Could you check a few things on this model? Use its own coordinates, in mm. A direction names the side the tool comes from. Coordinates: 2 decimals unless noted, no trailing zeros.
```python
from build123d import *

# Parameters (mm, degrees)
BOX001_W        = 38.73
BOX001_H        = 53.34
BOX001_DEPTH    = 50.8
SKETCH_W        = 139.7
SKETCH_H        = 127
SKETCH_W_2      = 130.175
SKETCH_H_2      = 115.8875
PAD_DEPTH       = 31.75
SKETCH001_W     = 139.7
SKETCH001_H     = 127
SKETCH001_R     = 1.651
PAD001_DEPTH    = 4.7625
SKETCH002_R     = 5.08
SKETCH002_R_2   = 2.286
PAD002_DEPTH    = 31.75
SKETCH003_W     = 25.4
SKETCH003_H     = 40
PAD003_DEPTH    = 24.5
POCKET_DEPTH    = 139.701
SKETCH007_R     = 4.445
SKETCH007_R_2   = 1.45
PAD006_DEPTH    = 6.35
SKETCH014_R     = 1.905
POCKET004_DEPTH = 6.351
SKETCH015_W     = 133.35
SKETCH015_H     = 120.65
POCKET005_DEPTH = 6.35
SKETCH016_R     = 1.651
PAD010_DEPTH    = 3.175
SKETCH060_W     = 10.16
SKETCH060_H     = 9.525
SKETCH060_W_2   = 7.62
SKETCH060_H_2   = 1.143
PAD028_DEPTH    = 9.525
SKETCH061_R     = 1.6
POCKET028_DEPTH = 11.43
SKETCH071_W     = 4.522567
SKETCH071_H     = 19.0781560115
PAD033_DEPTH    = 28.575
SKETCH072_R     = 1.778
POCKET034_DEPTH = 76.2
SKETCH074_W     = 4.299609
SKETCH074_H     = 32.990636
SKETCH074_W_2   = 34.861665
SKETCH074_H_2   = 4.058911
PAD034_DEPTH    = 28.575
SKETCH089_W     = 5.08
SKETCH089_H     = 47.5033603219
SKETCH089_R     = 1.45
PAD041_DEPTH    = 19.05


with BuildPart() as front_removal:
    # Box001 → Box001 (new body)
    with BuildSketch(Plane(origin=(-14.6558, 22.7838, 0), x_dir=(1, 0, 0), z_dir=(0, 0, 1))):
        with Locations((19.365, 26.67)):
            Rectangle(BOX001_W, BOX001_H)
    extrude(amount=BOX001_DEPTH)


with BuildPart() as main_body:
    # Sketch → Pad (new body)
    with BuildSketch(Plane.XY):
        Rectangle(SKETCH_W, SKETCH_H)
        with Locations((0, -0.79375)):
            Rectangle(SKETCH_W_2, SKETCH_H_2, mode=Mode.SUBTRACT)
    extrude(amount=PAD_DEPTH)

    # Sketch001 (on Face9 of Pad) → Pad001 (join)
    with BuildSketch(Plane(origin=(0, 0, 0), x_dir=(1, 0, 0), z_dir=(0, 0, -1))):
        Rectangle(SKETCH001_W, SKETCH001_H)
        with Locations((-27.286566, 13.226975)):
            Circle(SKETCH001_R, mode=Mode.SUBTRACT)
        with Locations((-27.286566, -2.648025)):
            Circle(SKETCH001_R, mode=Mode.SUBTRACT)
        with Locations((-9.8298, -32.495678)):
            Circle(SKETCH001_R, mode=Mode.SUBTRACT)
        with Locations((19.2024, -32.495678)):
            Circle(SKETCH001_R, mode=Mode.SUBTRACT)
        with Locations((19.2024, -56.625678)):
            Circle(SKETCH001_R, mode=Mode.SUBTRACT)
        with Locations((-9.8298, -56.625678)):
            Circle(SKETCH001_R, mode=Mode.SUBTRACT)
    extrude(amount=PAD001_DEPTH)

    # Sketch002 (on Face21 of Pad001) → Pad002 (join)
    with BuildSketch(Plane.XY):
        with Locations((-62.70625, 55.5625)):
            Circle(SKETCH002_R)
        with Locations((-62.70625, 55.5625)):
            Circle(SKETCH002_R_2, mode=Mode.SUBTRACT)
        with Locations((0, 55.5625)):
            Circle(SKETCH002_R)
        with Locations((0, 55.5625)):
            Circle(SKETCH002_R_2, mode=Mode.SUBTRACT)
        with Locations((62.70625, 55.5625)):
            Circle(SKETCH002_R)
        with Locations((62.70625, 55.5625)):
            Circle(SKETCH002_R_2, mode=Mode.SUBTRACT)
        with Locations((62.70625, 0)):
            Circle(SKETCH002_R)
        with Locations((62.70625, 0)):
            Circle(SKETCH002_R_2, mode=Mode.SUBTRACT)
        with Locations((62.70625, -55.5625)):
            Circle(SKETCH002_R)
        with Locations((62.70625, -55.5625)):
            Circle(SKETCH002_R_2, mode=Mode.SUBTRACT)
        with Locations((0, -55.5625)):
            Circle(SKETCH002_R)
        with Locations((0, -55.5625)):
            Circle(SKETCH002_R_2, mode=Mode.SUBTRACT)
        with Locations((-62.70625, -55.5625)):
            Circle(SKETCH002_R)
        with Locations((-62.70625, -55.5625)):
            Circle(SKETCH002_R_2, mode=Mode.SUBTRACT)
        with Locations((-62.70625, 0)):
            Circle(SKETCH002_R)
        with Locations((-62.70625, 0)):
            Circle(SKETCH002_R_2, mode=Mode.SUBTRACT)
    extrude(amount=PAD002_DEPTH)

    # Sketch003 (on Face33 of Pad002) → Pad003 (join)
    with BuildSketch(Plane.XY):
        with Locations((-57.15, -33.97)):
            Rectangle(SKETCH003_W, SKETCH003_H)
        with Locations((57.15, -33.97)):
            Rectangle(SKETCH003_W, SKETCH003_H)
    extrude(amount=PAD003_DEPTH)

    # Sketch004 (on Face7 of Pad003) → Pocket (cut, through all)
    with BuildSketch(Plane(origin=(-69.85, 0, 0), x_dir=(0, -1, 0), z_dir=(-1, 0, 0))):
        with BuildLine():
            ThreePointArc((24.511, 20.5930335595), (34.036, 0), (43.561, 20.5930335595))
            Line((43.561, 33.2930335595), (43.561, 20.5930335595))
            Line((24.511, 33.2930335595), (43.561, 33.2930335595))
            Line((24.511, 20.5930335595), (24.511, 33.2930335595))
        make_face()
    extrude(amount=-POCKET_DEPTH, mode=Mode.SUBTRACT)

    # Sketch007 → Pad006 (join)
    with BuildSketch(Plane(origin=(-34.29, 25.4, 0), x_dir=(1, 0, 0), z_dir=(0, 0, 1))):
        with Locations((5.08, 23.11)):
            Circle(SKETCH007_R)
        with Locations((5.08, 23.11)):
            Circle(SKETCH007_R_2, mode=Mode.SUBTRACT)
        with Locations((-26.92, 23.11)):
            Circle(SKETCH007_R)
        with Locations((-26.92, 23.11)):
            Circle(SKETCH007_R_2, mode=Mode.SUBTRACT)
        with Locations((-26.92, -8.89)):
            Circle(SKETCH007_R)
        with Locations((-26.92, -8.89)):
            Circle(SKETCH007_R_2, mode=Mode.SUBTRACT)
        with Locations((5.08, -8.89)):
            Circle(SKETCH007_R)
        with Locations((5.08, -8.89)):
            Circle(SKETCH007_R_2, mode=Mode.SUBTRACT)
    extrude(amount=PAD006_DEPTH)

    # Sketch014 (on Face19 of Pad006) → Pocket004 (cut, through all)
    with BuildSketch(Plane.XZ.offset(-57.15)):
        with Locations((-47.625, 21.59)):
            Circle(SKETCH014_R)
        with Locations((-28.575, 15.24)):
            Circle(SKETCH014_R)
        with Locations((33.655, 15.24)):
            Circle(SKETCH014_R)
        with Locations((52.705, 21.59)):
            Circle(SKETCH014_R)
    extrude(amount=-POCKET004_DEPTH, mode=Mode.SUBTRACT)

    # Sketch015 → Pocket005 (cut)
    with BuildSketch(Plane.XY.offset(29.21)):
        Rectangle(SKETCH015_W, SKETCH015_H)
    extrude(amount=POCKET005_DEPTH, mode=Mode.SUBTRACT)

    # Sketch016 (on Face11 of Pocket005) → Pad010 (join)
    with BuildSketch(Plane(origin=(-69.85, 0, 0), x_dir=(0, -1, 0), z_dir=(-1, 0, 0))):
        with BuildLine():
            ThreePointArc((30.226, 12.3860423935), (34.036, 8.5760423935), (37.846, 12.3860423935))
            Line((43.561, 20.5930335595), (37.846, 12.3860423935))
            ThreePointArc((24.511, 20.5930335595), (34.036, -0.1869576065), (43.561, 20.5930335595))
            Line((24.511, 20.5930335595), (30.226, 12.3860423935))
        make_face()
        with Locations((25.536, 12.49934)):
            Circle(SKETCH016_R, mode=Mode.SUBTRACT)
        with Locations((42.536, 12.49934)):
            Circle(SKETCH016_R, mode=Mode.SUBTRACT)
    pad010 = extrude(amount=-PAD010_DEPTH)

    # Mirrored: Pad010 across YZ
    add(pad010.mirror(Plane.YZ))

    # Sketch060 (on Face81 of Pocket005) → Pad028 (join)
    with BuildSketch(Plane.XY):
        with Locations((17.78, -53.975)):
            Rectangle(SKETCH060_W, SKETCH060_H)
        with Locations((17.78, -52.2605)):
            Rectangle(SKETCH060_W_2, SKETCH060_H_2, mode=Mode.SUBTRACT)
        with Locations((17.78, -56.5785)):
            Rectangle(SKETCH060_W_2, SKETCH060_H_2, mode=Mode.SUBTRACT)
    extrude(amount=PAD028_DEPTH)

    # Sketch061 (on Face86 of Pad028) → Pocket028 (cut)
    with BuildSketch(Plane.XZ.offset(63.5)):
        with Locations((17.78, 5.08)):
            Circle(SKETCH061_R)
    extrude(amount=-POCKET028_DEPTH, mode=Mode.SUBTRACT)

    # Sketch071 (on Face21 of Pad001) → Pad033 (join)
    with BuildSketch(Plane.XY):
        with Locations((-16.9815035, 50.9765749943)):
            Rectangle(SKETCH071_W, SKETCH071_H)
        with Locations((26.3779375001, 50.9765749943)):
            Rectangle(SKETCH071_W, SKETCH071_H)
    extrude(amount=PAD033_DEPTH)

    # Sketch072 (on Face127 of Pad033) → Pocket034 (cut)
    with BuildSketch(Plane.XY.offset(31.75)):
        with Locations((50.8, 22.225)):
            Circle(SKETCH072_R)
    extrude(amount=-POCKET034_DEPTH, mode=Mode.SUBTRACT)

    # Sketch074 (on Face56 of Pocket034) → Pad034 (join)
    with BuildSketch(Plane.XY):
        with Locations((-17.2816815, 25.842361)):
            Rectangle(SKETCH074_W, SKETCH074_H)
        with Locations((2.0425745, -22.9079595)):
            Rectangle(SKETCH074_W_2, SKETCH074_H_2)
    extrude(amount=PAD034_DEPTH)

    # Sketch089 (on Face56 of Pad034) → Pad041 (join)
    with BuildSketch(Plane.XY):
        with Locations((26.6647168511, 17.7529041609)):
            Rectangle(SKETCH089_W, SKETCH089_H)
        with Locations((26.6647168511, 32.117611)):
            Circle(SKETCH089_R, mode=Mode.SUBTRACT)
        with Locations((26.6647168511, 6.717611)):
            Circle(SKETCH089_R, mode=Mode.SUBTRACT)
    extrude(amount=PAD041_DEPTH)

    # Cut001: cut front-removal
    add(front_removal.part, mode=Mode.SUBTRACT)


solid = main_body.part
```
Item 1: Thinking about a two-plate mould opening in Y: for faces 1 (the face through (-10.188, 58.237, -2.348)), 2 (the face through (-67, 33, 31.75)), which applies, +Y half, -Y half, draft (parallel to the pull), parting line (faces both ways), or undercut?
Item 2: I need wall thicknesses on line 1 (X direction, y = 31, z = 23.5); line 2 (X direction, y = 28, z = 4); line 3 (Y direction, x = -22.5, z = 5). Which ranges of each line are inside material? Lowest first, please.
Item 3: For pin 1 Ø1 at (x, z) = (-2, 8.5) entering from +Y; pin 2 Ø1.7 at (x, y) = (26.66, 6.72) entering from +Z; pin 3 Ø3.5 at (x, y) = (-62.71, 55.56) entering from +Z, each with a flat end and sliding along its axis, tell me the tip position at first contact or that it passes through.
Item 4: Which directions (+Z, -Z, +X, -X, +Y, -Y) give clear straight access to the entire face, cutting with the end or side of a thin tool? Please do faces 3 (the face through (16, -57.15, 5)), 4 (the face through (-60, -43.561, 24)), 5 (the face through (16.6, -54.44, 6.16)), 6 (the face through (66.675, -34, 8)), 7 (the face through (-10.188, 34.107, -2.348)).
Geometry results:
1. face 1: undercut
1. face 2: draft
2. line 1: x = -69.85 to -65.09, -19.43 to -15.13, 65.09 to 69.85
2. line 2: x = -69.85 to -65.09, -19.43 to -15.13, 24.12 to 29.2, 65.09 to 69.85
2. line 3: y = -63.5 to -58.74, 57.15 to 63.5
3. pin 1: stops at y = -20.88
3. pin 2: stops at z = 0
3. pin 3: stops at z = 29.21
4. face 3: +Z
4. face 4: +Z, +X, -X
4. face 5: -Y
4. face 6: none
4. face 7: +Z, -Z
